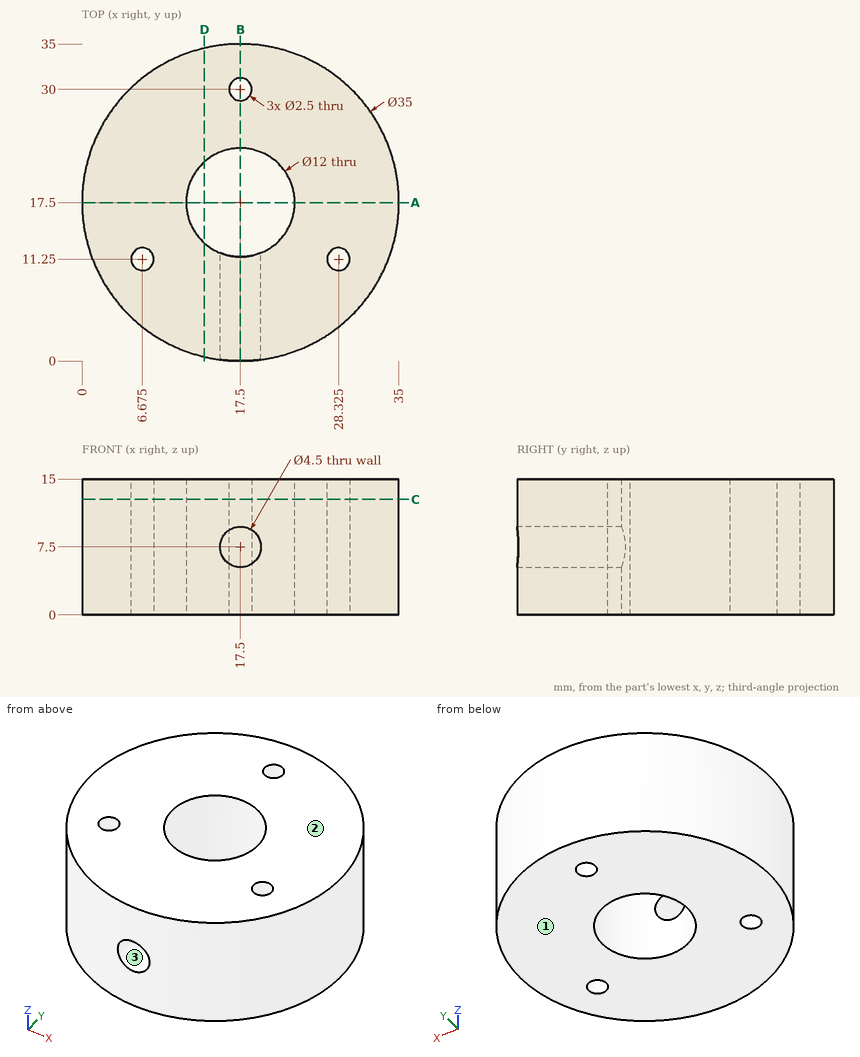
Answer from the drawing. Dimensions are ordinates in mm from the lowest x, y and z of the part. Give positions to 0.01 mm unless a question says otherwise; leave off trailing zeros. Order: outer loops, then holes, each group sorted by start corner. A loop starts at its lowest first (then second) coordinate and runs counter-clockwise, first axis right, second up.
(1) Given pin 1 (1.5 mm diameter, centred on x = 6.67, y = 11.25, fed in from -Z); pin 2 (4 mm diameter, centred on y = 15, z = 4.5, fed in from +X); pin 3 (4 mm diameter, centred on x = 11.5, z = 7, fed in from +Y); pin 4 (1 mm diameter, centred on y = 10, z = 10, fed in from +X), each flat-ended and moving along its own axis, determine where each tip first touches the part or whether it passes through.
(2) Find section C-C (z = 12.75). Give the number of separate pieces and of enclosed holes in the cut face, plus the area to 3 significant figures.
(3) Straight lines are drawn through the part: L1, parallel to X at y = 12, z = 9 (1 decimal); L2, parallel to Z at x = 19, y = 9; L3, parallel to X at y = 19, z = 1.5 (1 decimal). For each, find the intervals that lie inside material, in ascending order.
(4) Find section D-D (x = 13.5). Give the vertices of the cut face in (y, z), plus the area to 3 significant figures.
(5) Find section A-A (y = 17.5). Give the vertices of the cut face in (x, z).
(6) Find section B-B (x = 17.5). Give the vertices of the cut face in (y, z).
(7) For a pull along Z with two mould halves and no side action, classify the marked faces 1, 2 and 3 as released by +Z, released by -Z, zero draft, split by the parting line, or undercut.
Result sheet:
1. pin 1: passes through
1. pin 2: stops at x = 34.99
1. pin 3: stops at y = 34.54
1. pin 4: stops at x = 33.54
2. separate pieces: 1
2. enclosed holes: 4
2. area: 834 mm2
3. L1: x = 0.9 to 5.7, 7.7 to 15.1, 19.9 to 27.3, 29.3 to 34.1
3. L2: z = 0 to 5.82, 9.18 to 15
3. L3: x = 0.1 to 11.7, 23.3 to 34.9
4. outline: (0.46, 0) - (13.03, 0) - (13.03, 15) - (0.46, 15) - close; (21.97, 0) - (34.54, 0) - (34.54, 15) - (21.97, 15) - close
4. area: 377 mm2
5. outline: (0, 0) - (11.5, 0) - (11.5, 15) - (0, 15) - close; (23.5, 0) - (35, 0) - (35, 15) - (23.5, 15) - close
6. outline: (0, 0) - (11.5, 0) - (11.5, 5.25) - (0, 5.25) - close; (0, 9.75) - (11.5, 9.75) - (11.5, 15) - (0, 15) - close; (23.5, 0) - (28.75, 0) - (28.75, 15) - (23.5, 15) - close; (31.25, 0) - (35, 0) - (35, 15) - (31.25, 15) - close
7. face 1: released by -Z
7. face 2: released by +Z
7. face 3: undercut
